Answer from the drawing. Dimensions are ordinates in mm from the lowest x, y and z of the part. Round coordinates to 2 decimals unless told otherwise and drop trailing zeros. Write each loop counter-clockwise with the first axis right and the second up, starting at its lowest first coordinate (ties: lowest second). Pieces come first, ordered by that corner, then holes. Notation, with made-up numbers: (74.5, -15.5) - (112.5, -15.5) arc R22 ccw to (112.5, 4.5) - close; hole circle Ø2 at (4.25, 62.5). An arc over 180 degrees is marked (long way). Use a Markdown table: item, result. Add a question column.
1) Each of these flat-tipped pins is pushed along its axis until it touches: P1, Ø8, axis at y = 7, z = 11, coming from the +X side; P2, Ø1.3, axis at x = 17.5, z = 2.5, coming from the -Y side; P3, Ø0.5, axis at x = 7.5, z = 2.5, coming from the +Y side. Where does it stop, or does it pass through?
2) A cutting plane is placed at A-A (z = 5.5). Give the vertices of the cut face in (x, y).
3) A cutting plane is placed at B-B (y = 10.5). Give the vertices of the cut face in (x, z).
4) A cutting plane is placed at D-D (z = 13). Give the vertices of the cut face in (x, y) (1 decimal), then the cut area to 3 significant figures.
5) Find the intervals of material crossed by probe 1 along Y at (x, z) = (12.75, 35.5); probe 2 along Z at (x, y) = (20.5, 10.75); probe 3 along Y at (x, z) = (8.5, 18.5), in increasing order. Write a range as from..to.
6) A cutting plane is placed at C-C (x = 5.75). Give the vertices of the cut face in (y, z) (1 decimal), then the cut area to 3 significant figures.
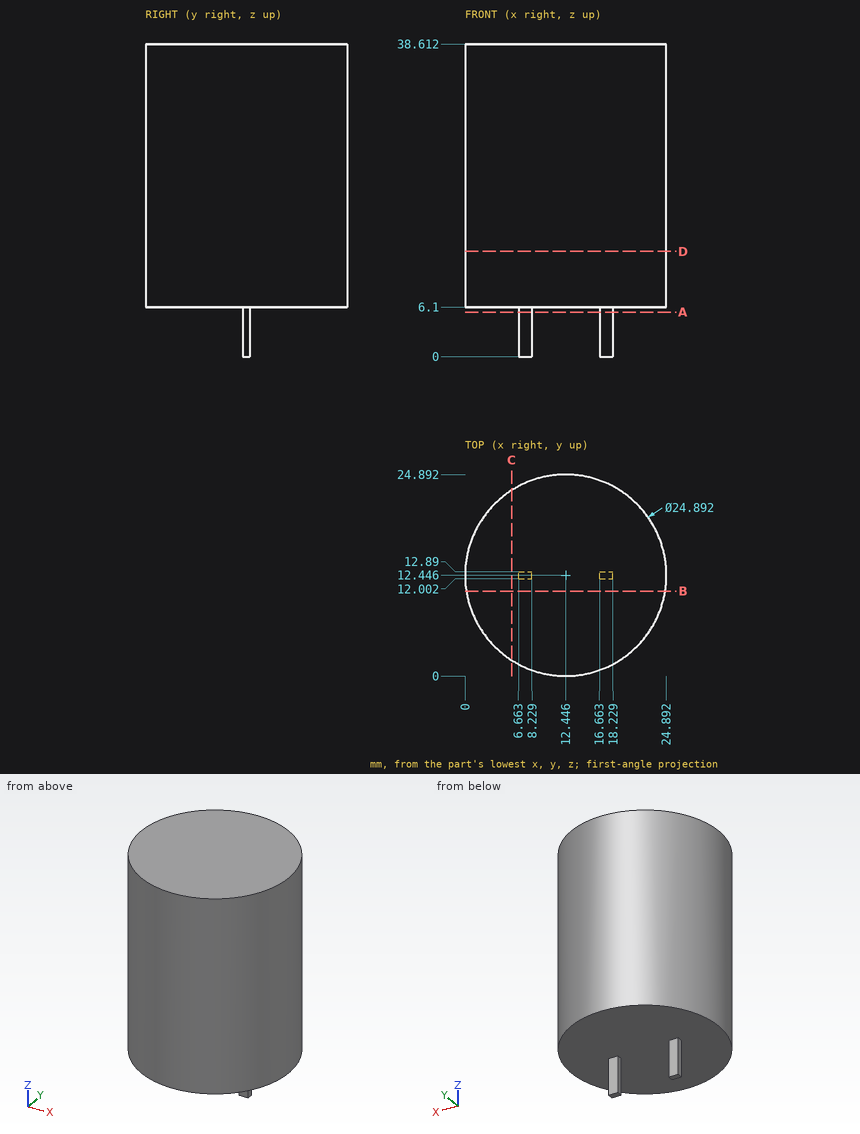
Entries:
| question | item | result |
|---|---|---|
| 1 | P1 | stops at x = 24.81 |
| 1 | P2 | stops at y = 12 |
| 1 | P3 | stops at y = 12.89 |
| 2 | outline | (6.66, 12) - (8.23, 12) - (8.23, 12.89) - (6.66, 12.89) - close; (16.66, 12) - (18.23, 12) - (18.23, 12.89) - (16.66, 12.89) - close |
| 3 | outline | (0.15, 6.1) - (24.74, 6.1) - (24.74, 38.61) - (0.15, 38.61) - close |
| 4 | outline | circle Ø24.9 at (12.4, 12.4) |
| 4 | area | 487 mm² |
| 5 | probe 1 | y = 0..24.89 |
| 5 | probe 2 | z = 6.1..38.61 |
| 5 | probe 3 | y = 0.64..24.25 |
| 6 | outline | (2, 6.1) - (22.9, 6.1) - (22.9, 38.6) - (2, 38.6) - close |
| 6 | area | 682 mm² |
